Can you work these out from the model? Positions are in its coordinate system, mm. A direction names the side the tool comes from. Round coordinates to 2 decimals unless told otherwise and drop trailing zeros. Loops run counter-clockwise (first coordinate to the right, second up) from the corner with the lowest first, then second, coordinate; pieces in that order, holes last. Notation, with made-up numbers: (74, 44.5) -> (111, 44.5) arc R20 cw to (111, 51.5) -> close; hole circle Ø3 at (-1, 63.5). An arc over 180 degrees is marked (long way). Use a Markdown table: item, result.
from build123d import *

# Parameters (mm, degrees)
F0_W     = 104
F0_H     = 44
F1_DEPTH = 4
F2_T     = -2
F4_DEPTH = 10


with BuildPart() as f1:
    # F0 (on Top) → F1 (new body)
    with BuildSketch(Plane.XY):
        with Locations((-52, 0)):
            Rectangle(F0_W, F0_H)
    extrude(amount=F1_DEPTH)

    # F2
    f2_openings = [f1.faces().sort_by_distance(p)[0] for p in [
        (-52, 0, 4),
    ]]
    offset(amount=F2_T, openings=f2_openings)

    # F3 (on face) → F4 (cut)
    with BuildSketch(Plane.XY):
        with BuildLine():
            Line((-82.539678, 22), (-21.460322, 22))
            ThreePointArc((-21.460322, 22), (-20.730103, 22.059424), (-20, 22.120252))
            Line((-20, 22.120252), (-20, 36.755234))
            Line((-20, 36.755234), (-84, 36.755234))
            Line((-84, 36.755234), (-84, 22.120252))
            ThreePointArc((-84, 22.120252), (-83.269897, 22.059424), (-82.539678, 22))
        make_face()
        with BuildLine():
            Line((-20, -36.755234), (-20, -22.120252))
            ThreePointArc((-20, -22.120252), (-20.730103, -22.059424), (-21.460322, -22))
            Line((-21.460322, -22), (-82.539678, -22))
            ThreePointArc((-82.539678, -22), (-83.269897, -22.059424), (-84, -22.120252))
            Line((-84, -22.120252), (-84, -36.755234))
            Line((-84, -36.755234), (-20, -36.755234))
        make_face()
    extrude(amount=F4_DEPTH, mode=Mode.SUBTRACT)


solid = f1.part
1. Will this pin go through, and if not, where does the flat tip stop? pin 1 Ø10 at (x, y) = (-78, -13) entering from +Z.
Answer sheet:
| item | result |
|---|---|
| pin 1 | stops at z = 2 |
2. I want a section at A-A (z = 3.1). Please give me the cut outline in (x, y), plus the area to 3 significant figures.
Answer sheet:
| item | result |
|---|---|
| outline | (-104, -22) -> (0, -22) -> (0, 22) -> (-104, 22) -> close; hole (-102, -20) -> (-2, -20) -> (-2, 20) -> (-102, 20) -> close |
| area | 576 mm² |
3. Which directions (+Z, -Z, +X, -X, +Y, -Y) give clear straight access to the entire face, cutting with the end or side of a thin tool? Please do faces 4 (the flat face through (-53, 0, 0)), 5 (the flat face through (-53, 20, 3)).
Answer sheet:
| item | result |
|---|---|
| face 4 | -Z, +X, -X, +Y, -Y |
| face 5 | +Z |
4. If we mould it in two halves opening along X, with no side actions, what happens to faces 1 (the flat face through (-102, 0, 3)), 2 (the flat face through (-68, -21, 4)), 3 (the flat face through (-104, 0, 2))? For each: +X half, -X half, draft (parallel to the pull), parting line (faces both ways), or undercut.
Answer sheet:
| item | result |
|---|---|
| face 1 | undercut |
| face 2 | draft |
| face 3 | -X half |
5. I need wall thicknesses on line 1 (Y direction, x = -42.5, z = 3.5); line 2 (X direction, y = 10.5, z = 2.55); line 3 (Z direction, x = -11.5, y = -5.5). Which ranges of each line are inside material? Lowest first, please.
Answer sheet:
| item | result |
|---|---|
| line 1 | y = -22 to -20, 20 to 22 |
| line 2 | x = -104 to -102, -2 to 0 |
| line 3 | z = 0 to 2 |
6. I want a section at B-B (y = -8.5). Please give me the cut outline in (x, z).
Answer sheet:
| item | result |
|---|---|
| outline | (-104, 0) -> (0, 0) -> (0, 4) -> (-2, 4) -> (-2, 2) -> (-102, 2) -> (-102, 4) -> (-104, 4) -> close |
7. I want a section at C-C (x = -92). Please give me the cut outline in (y, z).
Answer sheet:
| item | result |
|---|---|
| outline | (-22, 0) -> (22, 0) -> (22, 4) -> (20, 4) -> (20, 2) -> (-20, 2) -> (-20, 4) -> (-22, 4) -> close |
